The figure shows three views and two pictorial views of one solid part (mm, origin at its lowest corner). Answer the questions. A direction names the side the tool comes from. Round coordinates to 2 decimals unless told otherwise and drop trailing zeros. Order: outer loops, then holes, each group sorted by start corner. A loop starts at its lowest first (then second) coordinate and runs counter-clockwise, first axis right, second up. Notation, with made-up numbers: (24.25, 75.5) - (37.25, 75.5) arc R33 cw to (37.25, 113.5) - close; hole circle Ø9 at (14.5, 85). An arc over 180 degrees is marked (long way). Answer as a JSON object with one key per item and string values. Group by question number.
Q1. A cutting plane is placed at C-C on x = 17.5. Count the separate pieces of the cut face and the enclosed holes in it.
Q2. A cutting plane is placed at D-D on x = 11. Determine the outline of the cut face in (y, z).
Q3. A cutting plane is placed at B-B on y = 21. Determine the outline of the cut face in (x, z) (1 decimal), and give its area (3 significant figures).
Q4. Given pin 1 Ø6 at (x, y) = (6.5, 5) entering from -Z; pin 2 Ø7 at (x, z) = (7, 7) entering from +Y, each flat-ended and moving along its own axis, determine where each tip first touches the part or whether it passes through.
Q5. Consider line 1 (Y direction, x = 23.25, z = 5.75); line 2 (Z direction, x = 2, y = 12.5); line 3 (Y direction, x = 17, z = 24.25). Determine where each line is inside the solid, lowest interval first.
Q6. A cutting plane is placed at A-A on z = 12.7. Determine the outline of the cut face in (x, y) (1 decimal).
Q7. A tool of negligible diameter and unlimited length cuts with its end or side. For the marked faces 1 and 2, from which of +Z, -Z, +X, -X, +Y, -Y can it reach the whole face along a straight path? Write none if from no direction.
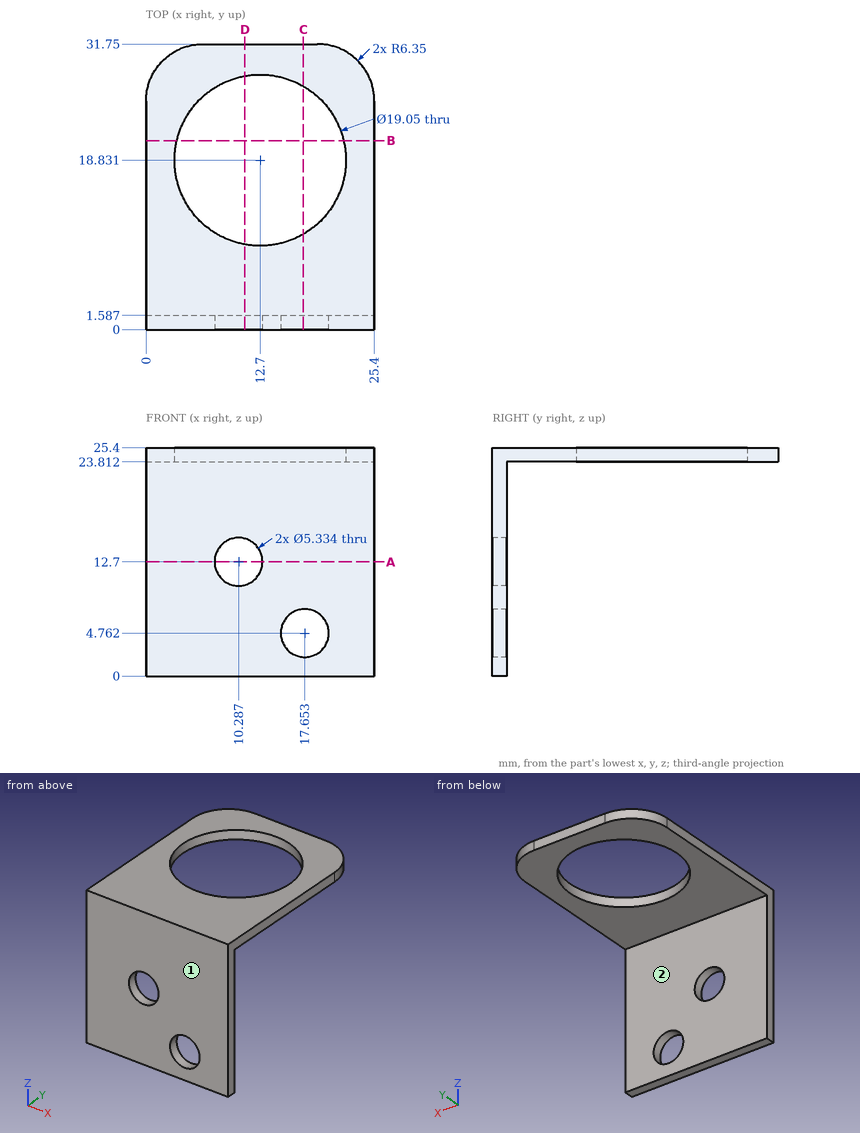
Result set:
{
 "1": {"separate pieces": "3", "enclosed holes": "0"},
 "2": {"outline": "(0, 0) - (1.59, 0) - (1.59, 10.13) - (0, 10.13) - close; (0, 15.27) - (1.59, 15.27) - (1.59, 23.81) - (9.46, 23.81) - (9.46, 25.4) - (0, 25.4) - close; (28.2, 23.81) - (31.75, 23.81) - (31.75, 25.4) - (28.2, 25.4) - close"},
 "3": {"outline": "(0, 23.8) - (3.4, 23.8) - (3.4, 25.4) - (0, 25.4) - close; (22, 23.8) - (25.4, 23.8) - (25.4, 25.4) - (22, 25.4) - close", "area": "10.9 mm²"},
 "4": {"pin 1": "stops at z = 23.81", "pin 2": "stops at y = 1.59"},
 "5": {"line 1": "y = 0 to 1.59", "line 2": "z = 23.81 to 25.4", "line 3": "y = 0 to 10.33, 27.33 to 31.75"},
 "6": {"outline": "(0, 0) - (7.6, 0) - (7.6, 1.6) - (0, 1.6) - close; (13, 0) - (25.4, 0) - (25.4, 1.6) - (13, 1.6) - close"},
 "7": {"face 1": "+Z, -Z, +X, -X, -Y", "face 2": "-Z, +X, -X, +Y"}
}
